Geometry check sheet. Reference: drawing and pictorial views, mm from the part's lowest x, y, z. A direction names the side the tool comes from. Coordinates: 2 decimals unless noted, no trailing zeros. Write each loop counter-clockwise with the first axis right and the second up, starting at its lowest first coordinate (ties: lowest second). Pieces come first, ordered by that corner, then holes. Notation, with made-up numbers: (-6, 32) - (9, 32) arc R36 cw to (9, 69) - close; hole circle Ø5 at (87, 6). An arc over 180 degrees is marked (long way). Answer as a JSON object with one key per item and string values. Group by question number.
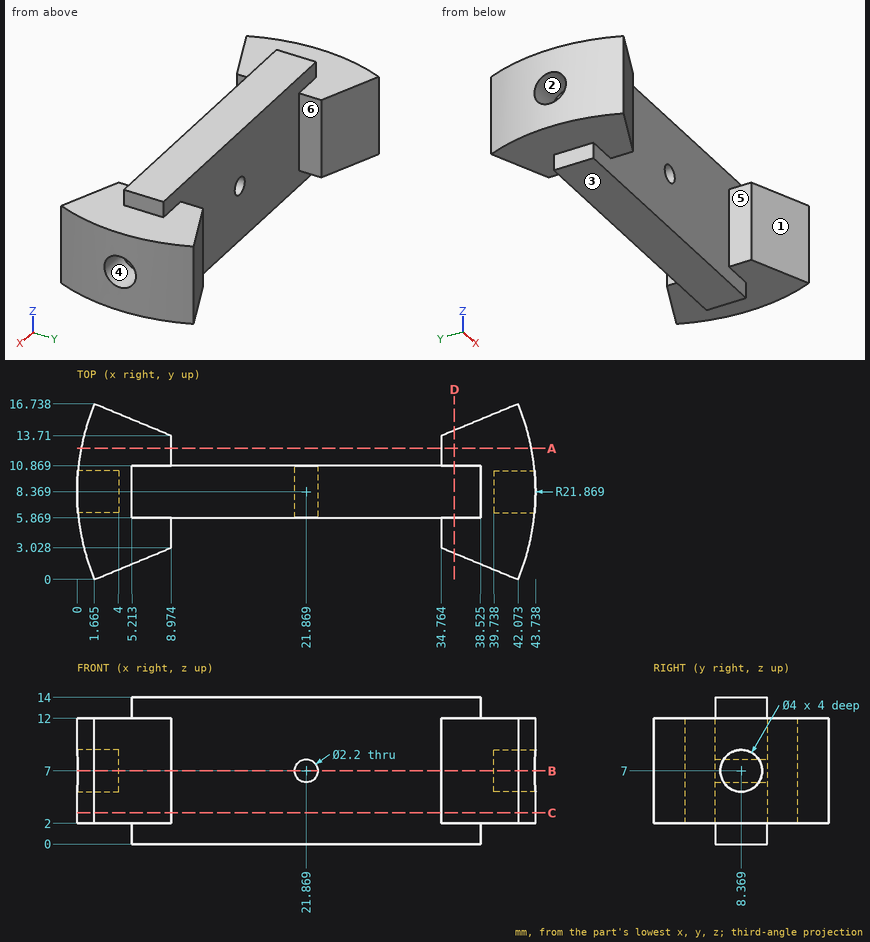
(1) Section check B-B (z = 7). Record the cut outline in (x, y) (1 decimal), and give its area (3 significant figures).
(2) Set-up check for the marked faces 4, 5 and 6: record each of +Z, -Z, +X, -X, +Y, -Y from which the full face is reachable in a straight line by a thin tool's end or side.
(3) Draft check along Y on the marked faces 1, 2 and 3. Enter one of: +Y half, -Y half, draft (parallel to the pull), parting line (faces both ways), or undercut.
(4) Gauge pin test, flat ends, axial feed: pin 1 (0.9 mm diameter, centred on y = 4, z = 4.5, fed in from -X); pin 2 (1.5 mm diameter, centred on x = 8.5, z = 9, fed in from +Y); pin 3 (0.9 mm diameter, centred on y = 12.5, z = 8, fed in from +X). Record the tip position at first contact, or that the pin passes through.
(5) Section check A-A (y = 12.5). Record the cut outline in (x, z) (1 decimal).
(6) Section check D-D (x = 36). Record the cut outline in (y, z) (1 decimal), and give its area (3 significant figures).
(7) Material ranges on L1, parallel to X at y = 6.9, z = 7; L2, parallel to X at y = 10.25, z = 1.5 (1 decimal); L3, parallel to Y at x = 3.15, z = 7 (1 decimal), recorded low to high. Write a range as [from, to].
(8) Section check C-C (z = 3). Record the cut outline in (x, y) (1 decimal), and give its area (3 significant figures).
Conclusion:
{
 "1": {"outline": "(0.1, 6.4) arc R21.9 ccw to (1.7, 0) - (9, 3) - (9, 5.9) - (20.8, 5.9) - (20.8, 10.9) - (9, 10.9) - (9, 13.7) - (1.7, 16.7) arc R21.9 ccw to (0.1, 10.4) - (4, 10.4) - (4, 6.4) - close; (23, 5.9) - (34.8, 5.9) - (34.8, 3) - (42.1, 0) arc R21.9 ccw to (43.6, 6.4) - (39.7, 6.4) - (39.7, 10.4) - (43.6, 10.4) arc R21.9 ccw to (42.1, 16.7) - (34.8, 13.7) - (34.8, 10.9) - (23, 10.9) - close", "area": "324 mm^2"},
 "2": {"face 4": "+X", "face 5": "+Z, -Z, -Y", "face 6": "+Z, -Z, +Y"},
 "3": {"face 1": "-Y half", "face 2": "undercut", "face 3": "draft"},
 "4": {"pin 1": "stops at x = 0.35", "pin 2": "stops at y = 14.22", "pin 3": "stops at x = 43.43"},
 "5": {"outline": "(0.4, 2) - (9, 2) - (9, 12) - (0.4, 12) - close; (34.8, 2) - (43.3, 2) - (43.3, 12) - (34.8, 12) - close"},
 "6": {"outline": "(2.5, 2) - (5.9, 2) - (5.9, 0) - (10.9, 0) - (10.9, 2) - (14.2, 2) - (14.2, 12) - (10.9, 12) - (10.9, 14) - (5.9, 14) - (5.9, 12) - (2.5, 12) - close", "area": "137 mm^2"},
 "7": {"L1": "x = [4, 20.77], [22.97, 39.74]", "L2": "x = [5.2, 38.5]", "L3": "y = [0.6, 6.4], [10.4, 16.1]"},
 "8": {"outline": "(1.7, 0) - (9, 3) - (9, 5.9) - (34.8, 5.9) - (34.8, 3) - (42.1, 0) arc R21.9 ccw to (42.1, 16.7) - (34.8, 13.7) - (34.8, 10.9) - (9, 10.9) - (9, 13.7) - (1.7, 16.7) arc R21.9 ccw to start", "area": "367 mm^2"}
}
